Part print with two shaded views. Sizes in mm from the minimum x, y, z corner. A direction names the side the tool comes from. Round coordinates to 2 decimals unless told otherwise and drop trailing zeros. Order: outer loops, then holes, each group sorted by start corner. A loop starts at its lowest first (then second) coordinate and runs counter-clockwise, first axis right, second up. Notation, with made-up numbers: (56.25, -13.5) -> (104.25, -13.5) arc R8 ccw to (104.25, 0.5) -> close; hole circle Ø4 at (9.25, -39). An arc over 180 degrees is marked (long way). Answer as a JSON object with one key per item and string values.
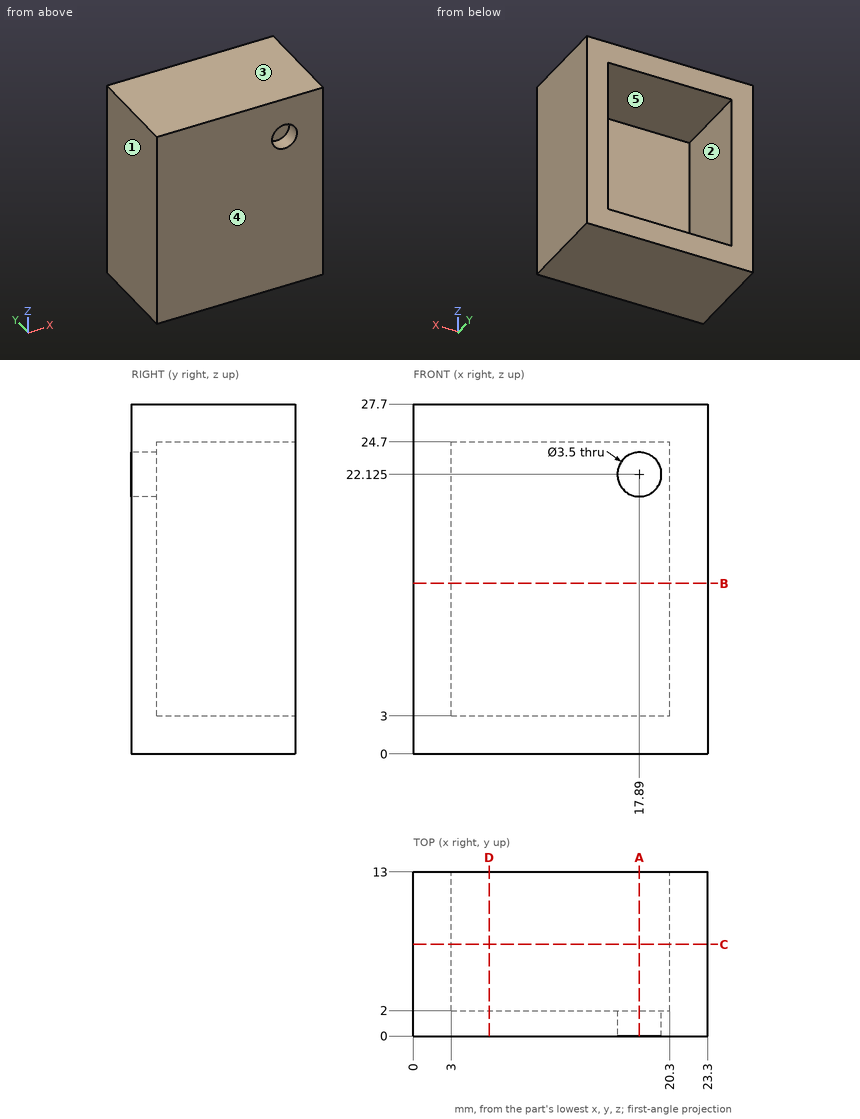
1) Cut at D-D, the plane x = 6. Give the cut face in (y, z).
Checked values:
{"outline": "(0, 0) -> (13, 0) -> (13, 3) -> (2, 3) -> (2, 24.7) -> (13, 24.7) -> (13, 27.7) -> (0, 27.7) -> close"}
2) Flat gauge pins, fed straight in: pin 1 Ø2 at (x, z) = (17.89, 22.13) entering from +Y; pin 2 Ø10 at (x, z) = (14, 15) entering from +Y. Where does each tip first touch, or does it go through?
Checked values:
{"pin 1": "passes through", "pin 2": "stops at y = 2"}
3) Cut at C-C, the plane y = 7.25. Give the cut face in (x, z).
Checked values:
{"outline": "(0, 0) -> (23.3, 0) -> (23.3, 27.7) -> (0, 27.7) -> close; hole (3, 3) -> (20.3, 3) -> (20.3, 24.7) -> (3, 24.7) -> close"}
4) Which spindle directions (+Z, -Z, +X, -X, +Y, -Y) get a long thin tool onto all of the face, cutting with end or side? Do the marked faces 4 and 5. Say none if no direction does.
Checked values:
{"face 4": "+Z, -Z, +X, -X, -Y", "face 5": "+Y"}
5) Cut at B-B, the plane z = 13.5. Give the cut face in (x, y).
Checked values:
{"outline": "(0, 0) -> (23.3, 0) -> (23.3, 13) -> (20.3, 13) -> (20.3, 2) -> (3, 2) -> (3, 13) -> (0, 13) -> close"}
6) Probe L1, parallel to Z at x = 7.5, y = 3.25; L2, parallel to X at y = 3, z = 11.5; L3, parallel to Z at x = 17.89, y = 1.3 (1 decimal). List the from-to ranges inside material, lowest first. Write a range as from..to.
Checked values:
{"L1": "z = 0..3, 24.7..27.7", "L2": "x = 0..3, 20.3..23.3", "L3": "z = 0..20.4, 23.9..27.7"}
7) Cut at A-A, the plane x = 17.89. Give the cut face in (y, z) (1 decimal).
Checked values:
{"outline": "(0, 0) -> (13, 0) -> (13, 3) -> (2, 3) -> (2, 20.4) -> (0, 20.4) -> close; (0, 23.9) -> (2, 23.9) -> (2, 24.7) -> (13, 24.7) -> (13, 27.7) -> (0, 27.7) -> close"}
8) Pull direction Z, two halves, no side cores. Call the marked faces 1, 2 and 3: pulls with the +Z half, pulls with the -Z half, needs draft (parallel to the pull), parting line crosses it, or undercut.
Checked values:
{"face 1": "needs draft", "face 2": "undercut", "face 3": "pulls with the +Z half"}
